The listing builds one solid part. Answer for the finished solid, in the listing's coordinates (mm). Face numbers are marked on the shaded views. A direction names the side the tool comes from. Give positions to 0.01 mm unless a question says otherwise; leave off trailing zeros. Loops run counter-clockwise (first coordinate to the right, second up) from the corner with the lowest first, then second, coordinate; pieces in that order, holes last. Notation, with made-up numbers: (-25.75, 21) - (-5.75, 21) arc R3 ccw to (-5.75, 25) - close; hole circle Ø11 at (48.5, -10.75). An arc over 180 degrees is marked (long way). Write each question's results on one line, items separated by ' | '.
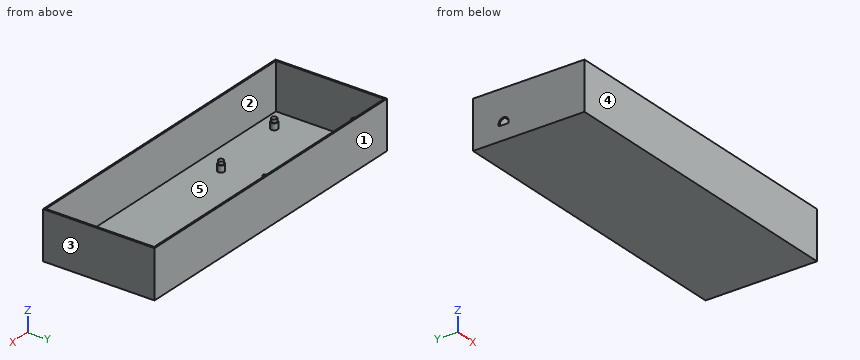
from build123d import *

# Parameters (mm, degrees)
F2_W     = 195.4786418714
F2_H     = 68
F2_R     = 2.1080985417
F2_R_2   = 2.1080985448
F2_R_3   = 2.1080987473
F2_R_4   = 2.1080985484
F3_DEPTH = 1
F2_R_5   = 1.6080985484
F2_R_6   = 1.6080987473
F2_R_7   = 1.6080985448
F2_R_8   = 1.6080985417
F4_DEPTH = 5
F5_DEPTH = 7
F2_H_2   = 1
F2_W_2   = 1
F6_DEPTH = 30
F8_DEPTH = 1


with BuildPart() as f3:
    # F2 (on Top) → F3 (new body)
    with BuildSketch(Plane.XY):
        with Locations((101.2606790643, 35)):
            Rectangle(F2_W, F2_H)
        with Locations((18.551614222, 11.0404381331)):
            Circle(F2_R, mode=Mode.SUBTRACT)
        with Locations((70.5820634049, 16.1186437591)):
            Circle(F2_R_2, mode=Mode.SUBTRACT)
        with Locations((70.5820629074, 44.0276153146)):
            Circle(F2_R_3, mode=Mode.SUBTRACT)
        with Locations((19.8211650697, 59.2622312398)):
            Circle(F2_R_4, mode=Mode.SUBTRACT)
    extrude(amount=F3_DEPTH)

    # F2 (on Top) → F4 (join)
    with BuildSketch(Plane.XY):
        with Locations((19.8211650697, 59.2622312398)):
            Circle(F2_R_4)
        with Locations((19.8211650697, 59.2622312398)):
            Circle(F2_R_5, mode=Mode.SUBTRACT)
        with Locations((70.5820629074, 44.0276153146)):
            Circle(F2_R_3)
        with Locations((70.5820629074, 44.0276153146)):
            Circle(F2_R_6, mode=Mode.SUBTRACT)
        with Locations((70.5820634049, 16.1186437591)):
            Circle(F2_R_2)
        with Locations((70.5820634049, 16.1186437591)):
            Circle(F2_R_7, mode=Mode.SUBTRACT)
        with Locations((18.551614222, 11.0404381331)):
            Circle(F2_R)
        with Locations((18.551614222, 11.0404381331)):
            Circle(F2_R_8, mode=Mode.SUBTRACT)
    extrude(amount=F4_DEPTH)

    # F2 (on Top) → F5 (join)
    with BuildSketch(Plane.XY):
        with Locations((19.8211650697, 59.2622312398)):
            Circle(F2_R_5)
        with Locations((70.5820629074, 44.0276153146)):
            Circle(F2_R_6)
        with Locations((70.5820634049, 16.1186437591)):
            Circle(F2_R_7)
        with Locations((18.551614222, 11.0404381331)):
            Circle(F2_R_8)
    extrude(amount=F5_DEPTH)

    # F2 (on Top) → F6 (join)
    with BuildSketch(Plane.XY):
        with Locations((101.2606790643, 69.5)):
            Rectangle(F2_W, F2_H_2)
        with Locations((199.5, 69.5)):
            Rectangle(F2_W_2, F2_H_2)
        Polygon((2.5213581286, 0), (3.5213581286, 0), (3.5213581286, 1), (3.5213581286, 69), (3.5213581286, 70), (2.5213581286, 70), align=None)
        with Locations((101.2606790643, 0.5)):
            Rectangle(F2_W, F2_H_2)
        with Locations((199.5, 0.5)):
            Rectangle(F2_W_2, F2_H_2)
        with Locations((199.5, 35)):
            Rectangle(F2_W_2, F2_H)
    extrude(amount=F6_DEPTH)

    # F7 (on face) → F8 (cut)
    with BuildSketch(Plane(origin=(2.5213581286, 0, 0), x_dir=(0, -1, 0), z_dir=(-1, 0, 0))):
        with BuildLine():
            Line((-53.966367571, 10.121377154), (-53.966367571, 9.9484939128))
            ThreePointArc((-53.966367571, 9.9484939128), (-53.9072548267, 9.4201302724), (-53.760526233, 8.9091183618))
            Line((-53.760526233, 8.9091183618), (-47.8451862662, 8.9091183618))
            ThreePointArc((-47.8451862662, 8.9091183618), (-47.6903499572, 9.4625889476), (-47.638164158, 10.0349355334))
            ThreePointArc((-47.638164158, 10.0349355334), (-50.7596314072, 13.1993324187), (-53.966367571, 10.121377154))
        make_face()
    extrude(amount=-F8_DEPTH, mode=Mode.SUBTRACT)


solid = f3.part
Item 1: Flat-ended cylindrical pins translate along their axes: P1, Ø2.5, axis at x = 71.5, y = 16, coming from the +Z side; P2, Ø20.5, axis at x = 114, y = 47.5, coming from the +Z side. Find the tip coordinate at first contact, or state that the pin passes through.
Values found:
P1: stops at z = 7 | P2: stops at z = 1
Item 2: For the marked faces 4 and 5, determine the directions among +Z, -Z, +X, -X, +Y, -Y from which every point of the face is accessible in a straight line to the end or side of a thin tool.
Values found:
face 4: +Z, -Z, +X, -X, -Y | face 5: +Z
Item 3: A cutting plane is placed at A-A, the plane z = 20.25. Determine the outline of the cut face in (x, y), plus the area to 3 significant figures.
Values found:
outline: (2.52, 0) - (200, 0) - (200, 70) - (2.52, 70) - close; hole (3.52, 1) - (199, 1) - (199, 69) - (3.52, 69) - close | area: 531 mm²
Item 4: A cutting plane is placed at B-B, the plane y = 31. Determine the outline of the cut face in (x, z), plus the area to 3 significant figures.
Values found:
outline: (2.52, 0) - (200, 0) - (200, 30) - (199, 30) - (199, 1) - (3.52, 1) - (3.52, 30) - (2.52, 30) - close | area: 255 mm²
Item 5: A cutting plane is placed at C-C, the plane x = 33. Determine the outline of the cut face in (y, z).
Values found:
outline: (0, 0) - (70, 0) - (70, 30) - (69, 30) - (69, 1) - (1, 1) - (1, 30) - (0, 30) - close
Item 6: For a pull along Y with two mould halves and no side action, classify the marked faces 1, 2 and 3 as released by +Y, released by -Y, zero draft, split by the parting line, or undercut.
Values found:
face 1: released by +Y | face 2: undercut | face 3: zero draft
Item 7: Find the intervals of material crossed by line 1 along X through (y, z) = (64, 22.75); line 2 along Y through (x, z) = (77.5, 19.5); line 3 along Z through (x, y) = (16.5, 32.5), in increasing order. Write a range as [from, to].
Values found:
line 1: x = [2.52, 3.52], [199, 200] | line 2: y = [0, 1], [69, 70] | line 3: z = [0, 1]
